```python
from build123d import *

# Parameters (mm, degrees)
ESQUISSE1_R           = 4
BOSS_EXTRU_1_DEPTH    = 81.5
ESQUISSE2_W           = 28
ESQUISSE2_H           = 1
ESQUISSE3_W           = 5
ESQUISSE3_H           = 1
TROU_TARAUD_M41_D     = 3.3
TROU_TARAUD_M41_DEPTH = 11.5
TROU_TARAUD_M41_TIP   = 0.991420021
TROU_TARAUD_M43_D     = 3.3
CHANFREIN1_SIZE       = 0.25


with BuildPart() as part:
    # Esquisse1 → Boss.-Extru.1 (new body)
    with BuildSketch(Plane.XY):
        Circle(ESQUISSE1_R)
    extrude(amount=BOSS_EXTRU_1_DEPTH)

    # Esquisse2 → Enlèvement de matière-Révolution1 (revolve, cut)
    with BuildSketch(Plane(origin=(0, 0, 0), x_dir=(0, 0, -1), z_dir=(1, 0, 0)), mode=Mode.PRIVATE) as enl_vement_de_mati_re_r_volution1_sk:
        with Locations((-14, 3.5)):
            Rectangle(ESQUISSE2_W, ESQUISSE2_H)
    revolve(enl_vement_de_mati_re_r_volution1_sk.sketch.rotate(Axis((0, 0, 0), (0, 0, 1)), 90), axis=Axis((0, 0, 0), (0, 0, 1)), mode=Mode.SUBTRACT)

    # Esquisse3 → Enlèvement de matière-Révolution2 (revolve, cut)
    with BuildSketch(Plane(origin=(0, 0, 0), x_dir=(0, 0, -1), z_dir=(1, 0, 0)), mode=Mode.PRIVATE) as enl_vement_de_mati_re_r_volution2_sk:
        with Locations((-79, 3.5)):
            Rectangle(ESQUISSE3_W, ESQUISSE3_H)
    revolve(enl_vement_de_mati_re_r_volution2_sk.sketch.rotate(Axis((0, 0, 81.5), (0, 0, -1)), 270), axis=Axis((0, 0, 81.5), (0, 0, -1)), mode=Mode.SUBTRACT)

    # Trou taraudé M41
    with Locations(Plane.XY.offset(81.5)):
        with Locations((0, 0)):
            Hole(TROU_TARAUD_M41_D / 2, depth=TROU_TARAUD_M41_DEPTH)
            with Locations((0, 0, -(TROU_TARAUD_M41_DEPTH + TROU_TARAUD_M41_TIP / 2))):  # 118° drill point
                Cone(0, TROU_TARAUD_M41_D / 2, TROU_TARAUD_M41_TIP, mode=Mode.SUBTRACT)

    # Trou taraudé M43 (through all)
    with Locations(Plane(origin=(0, 0, 0), x_dir=(-1, 0, 0), z_dir=(0, 0, -1))):
        with Locations((0, 0)):
            Hole(TROU_TARAUD_M43_D / 2)

    # Chanfrein1
    chanfrein1_edges = [part.edges().sort_by_distance(p)[0] for p in [
        (3, 0, 81.5),
        (3, 0, 76.5),
        (-4, 0, 76.5),
        (0, 1.65, 81.5),
        (-1.65, 0, 0),
        (3, 0, 0),
        (3, 0, 28),
        (-4, 0, 28),
    ]]
    chamfer(chanfrein1_edges, length=CHANFREIN1_SIZE)


solid = part.part
```
Verification items for the finished model (mm, model axes). A direction names the side the tool comes from. Coordinates: 2 decimals unless noted, no trailing zeros. Loops run counter-clockwise (first coordinate to the right, second up) from the corner with the lowest first, then second, coordinate; pieces in that order, holes last. Notation, with made-up numbers: (-8.75, 48.5) - (49.25, 48.5) arc R25 cw to (49.25, 78.5) - close; hole circle Ø11 at (17.5, 39.5). An arc over 180 degrees is marked (long way). Answer as a JSON object with one key per item and string values.
(1) Access from +Z, -Z, +X, -X, +Y, -Y to the whole of each face (thin tool, end or side, straight path). Record for faces 1 (the cylindrical face through (-0.867, -3.905, 51.914)), 2 (the flat face through (-1.4, 3.1, 76.5)), 3 (the flat face through (-1.4, -3.1, 28)).
Response:
{"face 1": "+Z, -Z", "face 2": "+Z", "face 3": "-Z"}
(2) Go/stop test with flat-tipped pins: pin 1 Ø1.5 at (x, z) = (3, 60) entering from +Y; pin 2 Ø3 at (x, y) = (0, 0) entering from +Z; pin 3 Ø1.5 at (x, y) = (-2, 3) entering from +Z. Record where each tip stops, or that it passes through.
Response:
{"pin 1": "stops at y = 3.31", "pin 2": "passes through", "pin 3": "stops at z = 81.39"}
(3) Cross-section at C-C, the plane z = 50. Record the boundary of the cut face in (x, y), then the cut area to 3 significant figures.
Response:
{"outline": "circle Ø8 at (0, 0); hole circle Ø3.3 at (0, 0)", "area": "41.7 mm²"}
(4) Scan lines: line 1 along Y through (x, z) = (0, 54.5); line 2 along Y through (x, z) = (0, 21). Record each from-to range of solid material in increasing order.
Response:
{"line 1": "y = -4 to -1.65, 1.65 to 4", "line 2": "y = -3 to -1.65, 1.65 to 3"}
(5) Cross-section at B-B, the plane z = 15.5. Record the boundary of the cut face in (x, y).
Response:
{"outline": "circle Ø6 at (0, 0); hole circle Ø3.3 at (0, 0)"}
